from build123d import *

# Parameters (mm, degrees)
SKIZZE1_W                       = 4
SKIZZE1_H                       = 5
AUFSATZ_LINEAR_AUSTRAGEN1_DEPTH = 115
VERRUNDUNG1_R                   = 1


with BuildPart() as part:
    # Skizze1 → Aufsatz-Linear austragen1 (new body)
    with BuildSketch(Plane(origin=(0, 0, 0), x_dir=(0, 0, -1), z_dir=(1, 0, 0))):
        with Locations((-1, -2.5)):
            Rectangle(SKIZZE1_W, SKIZZE1_H)
    extrude(amount=AUFSATZ_LINEAR_AUSTRAGEN1_DEPTH)

    # Verrundung1
    verrundung1_edges = [part.edges().sort_by_distance(p)[0] for p in [
        (57.5, -5, -1),
        (57.5, -5, 3),
    ]]
    fillet(verrundung1_edges, radius=VERRUNDUNG1_R)


solid = part.part
Geometry: final body of the model. Coordinates: model frame, mm. Round coordinates to 2 decimals unless told otherwise and drop trailing zeros. Order: outer loops, then holes, each group sorted by start corner. A loop starts at its lowest first (then second) coordinate and runs counter-clockwise, first axis right, second up.
Q1. Section A-A, the plane x = 105.5. Output: boundary loops of the cut face in (y, z), and give its area (3 significant figures).
Result sheet:
outline: (-5, 0) arc R1 ccw to (-4, -1) - (0, -1) - (0, 3) - (-4, 3) arc R1 ccw to (-5, 2) - close
area: 19.6 mm2
Q2. Material intervals for probe 1 along Y at (x, z) = (69.5, 2.8); probe 2 along Z at (x, y) = (43.5, -4.5); probe 3 along Y at (x, z) = (10, 2.4), sorted ascending.
Result sheet:
probe 1: y = -4.6 to 0
probe 2: z = -0.87 to 2.87
probe 3: y = -4.92 to 0
Q3. Mould query, pull axis Z, two halves, no side actions, for faces 1 (the face through (57, -2, 3)), 2 (the face through (57, -2, -1)), 3 (the face through (57, -5, 1)). Classes: released by +Z, released by -Z, zero draft, split by the parting line, or undercut.
Result sheet:
face 1: released by +Z
face 2: released by -Z
face 3: zero draft
